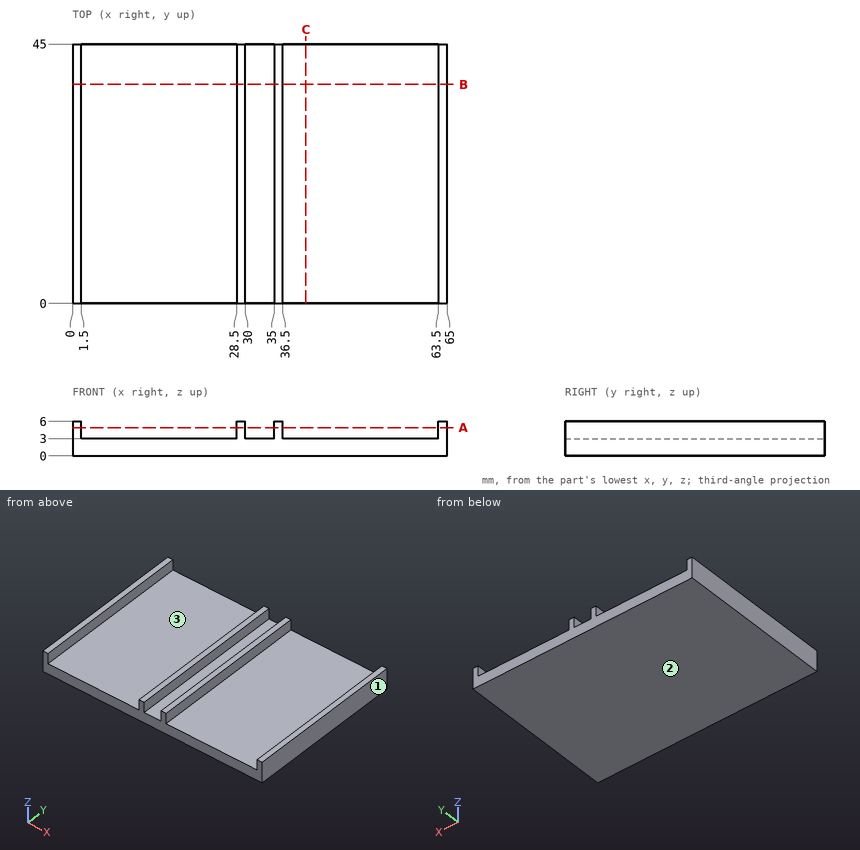
Print and shaded views of the part. All mm, measured from the part's lowest x, y and z. Coordinates: 2 decimals unless noted, no trailing zeros. Order: outer loops, then holes, each group sorted by start corner. A loop starts at its lowest first (then second) coordinate and runs counter-clockwise, first axis right, second up. Notation, with made-up numbers: (-17.75, 15) -> (36.25, 15) arc R11 cw to (36.25, 27) -> close; hole circle Ø11 at (65.5, -5.5). An arc over 180 degrees is marked (long way). Answer as a JSON object with one key per item and string values. Group by question number.
1) Cut at A-A, the plane z = 4.9. Write the cut outline in (x, y), then the cut area to 3 significant figures.
2) Cut at C-C, the plane x = 40.5. Write the cut outline in (y, z).
3) Flat gauge pin, fed straight in: pin 1 (4 mm diameter, centred on x = 32.5, y = 33, fed in from +Z). Where does the tip first touch, or does it go through?
4) Pull direction X, two halves, no side cores. Call the marked faces 1, 2 and 3: +X half, -X half, draft (parallel to the pull), parting line (faces both ways), or undercut.
5) Drill centre lines: L1, parallel to X at y = 16, z = 5.6; L2, parallel to Z at x = 24, y = 20. Where is each one in solid material? Low to high.
6) Cut at B-B, the plane y = 38. Write the cut outline in (x, z).
Check values:
{
 "1": {"outline": "(0, 0) -> (1.5, 0) -> (1.5, 45) -> (0, 45) -> close; (28.5, 0) -> (30, 0) -> (30, 45) -> (28.5, 45) -> close; (35, 0) -> (36.5, 0) -> (36.5, 45) -> (35, 45) -> close; (63.5, 0) -> (65, 0) -> (65, 45) -> (63.5, 45) -> close", "area": "270 mm²"},
 "2": {"outline": "(0, 0) -> (45, 0) -> (45, 3) -> (0, 3) -> close"},
 "3": {"pin 1": "stops at z = 3"},
 "4": {"face 1": "+X half", "face 2": "draft", "face 3": "undercut"},
 "5": {"L1": "x = 0 to 1.5, 28.5 to 30, 35 to 36.5, 63.5 to 65", "L2": "z = 0 to 3"},
 "6": {"outline": "(0, 0) -> (65, 0) -> (65, 6) -> (63.5, 6) -> (63.5, 3) -> (36.5, 3) -> (36.5, 6) -> (35, 6) -> (35, 3) -> (30, 3) -> (30, 6) -> (28.5, 6) -> (28.5, 3) -> (1.5, 3) -> (1.5, 6) -> (0, 6) -> close"}
}
